```python
from build123d import *

# Parameters (mm, degrees)
AUFSATZ_LINEAR_AUSTRAGEN1_DEPTH      = 45
AUFSATZ_LINEAR_AUSTRAGEN1_DEPTH_BACK = 45
SKIZZE3_W                            = 90
SKIZZE3_H                            = 65
SCHNITT_LINEAR_AUSTRAGEN1_DEPTH      = 120
SKIZZE4_R                            = 25
AUFSATZ_LINEAR_AUSTRAGEN2_DEPTH      = 20
SCHNITT_LINEAR_AUSTRAGEN2_DEPTH      = 65
SKIZZE6_W                            = 110
SKIZZE6_H                            = 30
SCHNITT_LINEAR_AUSTRAGEN3_DEPTH      = 120
SCHNITT_LINEAR_AUSTRAGEN4_DEPTH      = 30
SKIZZE8_R                            = 30
AUFSATZ_LINEAR_AUSTRAGEN3_DEPTH      = 15
VERRUNDUNG1_R                        = 20


with BuildPart() as part:
    # Skizze2 → Aufsatz-Linear austragen1 (new, two sides: drawn at the far end of the back side and taken through both)
    with BuildSketch(Plane(origin=(0, 0, 0), x_dir=(1, 0, 0), z_dir=(0, 1, 0)).offset(-AUFSATZ_LINEAR_AUSTRAGEN1_DEPTH_BACK)):
        with BuildLine():
            Line((-350, -60), (0, -60))
            ThreePointArc((0, -60), (60, 0), (0, 60))
            Line((0, 60), (-350, 60))
            ThreePointArc((-350, 60), (-410, 0), (-350, -60))
        make_face()
    extrude(amount=AUFSATZ_LINEAR_AUSTRAGEN1_DEPTH + AUFSATZ_LINEAR_AUSTRAGEN1_DEPTH_BACK)

    # Skizze3 → Schnitt-Linear austragen1 (cut)
    with BuildSketch(Plane.XY.offset(60)):
        with Locations((15, -12.5)):
            Rectangle(SKIZZE3_W, SKIZZE3_H)
    extrude(amount=-SCHNITT_LINEAR_AUSTRAGEN1_DEPTH, mode=Mode.SUBTRACT)

    # Skizze4 → Aufsatz-Linear austragen2 (add)
    with BuildSketch(Plane.XZ.offset(-20)):
        with Locations(Location((0, 0, 0), (0, 0, 180))):
            Circle(SKIZZE4_R)
    extrude(amount=AUFSATZ_LINEAR_AUSTRAGEN2_DEPTH)

    # Skizze5 → Schnitt-Linear austragen2 (cut)
    with BuildSketch(Plane.XZ.offset(45)):
        with BuildLine():
            Line((-30, 75), (-30, -75))
            ThreePointArc((-30, -75), (-105, 0), (-30, 75))
        make_face()
    extrude(amount=-SCHNITT_LINEAR_AUSTRAGEN2_DEPTH, mode=Mode.SUBTRACT)

    # Skizze6 → Schnitt-Linear austragen3 (cut)
    with BuildSketch(Plane.XY.offset(60)):
        with Locations((-355, -30)):
            Rectangle(SKIZZE6_W, SKIZZE6_H)
    extrude(amount=-SCHNITT_LINEAR_AUSTRAGEN3_DEPTH, mode=Mode.SUBTRACT)

    # Skizze7 → Schnitt-Linear austragen4 (cut)
    with BuildSketch(Plane(origin=(0, -45, 0), x_dir=(-1, 0, 0), z_dir=(0, -1, 0))):
        with BuildLine():
            Line((300, -60), (300, 60))
            ThreePointArc((300, 60), (240, 0), (300, -60))
        make_face()
    extrude(amount=-SCHNITT_LINEAR_AUSTRAGEN4_DEPTH, mode=Mode.SUBTRACT)

    # Skizze8 → Aufsatz-Linear austragen3 (add)
    with BuildSketch(Plane(origin=(0, -15, 0), x_dir=(-1, 0, 0), z_dir=(0, -1, 0))):
        with Locations(Location((350, 0, 0), (0, 0, 270))):
            Circle(SKIZZE8_R)
    extrude(amount=AUFSATZ_LINEAR_AUSTRAGEN3_DEPTH)

    # Verrundung1
    verrundung1_edges = [part.edges().sort_by_distance(p)[0] for p in [
        (-175, 45, 60),
        (-175, 45, -60),
        (-410, 45, 0),
        (60, 45, 0),
    ]]
    fillet(verrundung1_edges, radius=VERRUNDUNG1_R)


solid = part.part
```
Could you check a few things on this model? Use its own coordinates, in mm. A direction names the side the tool comes from. Give positions to 0.01 mm unless a question says otherwise; leave off trailing zeros. Loops run counter-clockwise (first coordinate to the right, second up) from the corner with the lowest first, then second, coordinate; pieces in that order, holes last. Notation, with made-up numbers: (31, -23) - (64, -23) arc R26 cw to (64, 14) - close; hole circle Ø5 at (-17.75, -6). An arc over 180 degrees is marked (long way). Answer in a Markdown table with one row per item. Add a question column.
Q1. We'd pull the mould along Z, two halves only. Please class faces 1 (the face through (-216, -10, 60)), 2 (the face through (-240.015, -30.21, -1.319)), 3 (the face through (59.985, 22.465, 1.319)): +Z half, -Z half, draft (parallel to the pull), parting line (faces both ways), or undercut.
Q2. If we section it at D-D (y = -23.5): List the corners of the cut face in (x, z) for me.
Q3. If we section it at B-B (y = 9.5): List the corners of the cut face in (x, z) for me.
Q4. For pin 1 (10 mm diameter, centred on y = 4.5, z = -42, fed in from +X); pin 2 (3 mm diameter, centred on y = 2.5, z = 11.5, fed in from +X); pin 3 (3 mm diameter, centred on x = -1.5, y = 28.5, fed in from +Z), each with a flat end and sliding along its axis, tell me the tip position at first contact or that it passes through.
Q5. If we section it at A-A (z = 0): List the corners of the cut face in (x, y) for me, plus the area to 3 significant figures.
Q6. Which directions (+Z, -Z, +X, -X, +Y, -Y) give clear straight access to the entire face, cutting with the end or side of a thin tool? Please do faces 4 (the face through (0, 0, 0)), 5 (the face through (-320.713, -22.395, -6.503)), 6 (the face through (-350, -30, 0)), 7 (the face through (-178, 45, -1)), 8 (the face through (-164, -45, -1)).
Q7. Please list where these lines run through material, in increasing order: L1, parallel to Z at x = -171, y = 25.5; L2, parallel to X at y = 17.5, z = 18.5; L3, parallel to X at y = 5.5, z = -9.5. Write a range as from..to.
Q8. If we section it at C-C (x = -264): List the corners of the cut face in (y, z) for me, plus the area to 3 significant figures.
The answers:
| question | item | result |
|---|---|---|
| 1 | face 1 | +Z half |
| 1 | face 2 | undercut |
| 1 | face 3 | parting line |
| 2 | outline | circle Ø60 at (-350, 0); (-300, -60) - (-75, -60) arc R75 cw to (-75, 60) - (-300, 60) arc R60 cw to start |
| 3 | outline | (-350, -60) - (-75, -60) arc R75 cw to (-75, 60) - (-350, 60) arc R60 ccw to start; circle Ø50 at (0, 0) |
| 4 | pin 1 | stops at x = -88.45 |
| 4 | pin 2 | stops at x = 22.91 |
| 4 | pin 3 | stops at z = 59.9 |
| 5 | outline | (-410, -15) - (-380, -15) - (-380, -30) - (-320, -30) - (-320, -15) - (-240, -15) - (-240, -45) - (-105, -45) - (-105, 20) - (-25, 20) - (-25, 0) - (25, 0) - (25, 20) - (60, 20) - (60, 25) arc R20 ccw to (40, 45) - (-390, 45) arc R20 ccw to (-410, 25) - close |
| 5 | area | 28,200 mm^2 |
| 6 | face 4 | +Z, -Z, +X, -Y |
| 6 | face 5 | -Y |
| 6 | face 6 | +Z, -Z, -X, -Y |
| 6 | face 7 | +Z, -Z, +X, -X, +Y |
| 6 | face 8 | +Z, -Z, +X, -X, -Y |
| 7 | L1 | z = -59.99..59.99 |
| 7 | L2 | x = -407.08..-102.68, -16.82..16.82 |
| 7 | L3 | x = -409.24..-104.4, -23.12..23.12 |
| 8 | outline | (-45, -60) - (25, -60) arc R20 ccw to (45, -40) - (45, 40) arc R20 ccw to (25, 60) - (-45, 60) - (-45, 48) - (-15, 48) - (-15, -48) - (-45, -48) - close |
| 8 | area | 7,750 mm^2 |
